from build123d import *

# Parameters (mm, degrees)
F2_R = 0.99999


# Not quite as in the source:
# - a fillet or chamfer is up to 0.001 mm smaller than in the source, because OpenCascade refuses the exact size


with BuildPart() as f1:
    # F0 (on Front) → F1 (revolve)
    with BuildSketch(Plane.XZ):
        with BuildLine():
            Line((-64.5, 52), (-65.5, 52))
            Line((-65.5, 52), (-65.5, 73))
            Line((-65.5, 73), (-67.5, 73))
            Line((-67.5, 73), (-67.5, 50))
            Line((-67.5, 50), (-66.1449700482, 50))
            ThreePointArc((-66.1449700482, 50), (-53.4398255255, 22.2737739938), (-30, 2.761242502))
            Line((-30, 2.761242502), (-30, -2))
            Line((-30, -2), (0, -2))
            Line((0, -2), (0, 0))
            Line((0, 0), (-28, 0))
            Line((-28, 0), (-28, 4))
            ThreePointArc((-28, 4), (-51.9728387009, 23.6482580712), (-64.5, 52))
        make_face()
    revolve(axis=Axis((0, 0, -1), (0, 0, -1)))

    # F2 (radius 1 in the source; OpenCascade refuses exactly that, so slightly less here)
    f2_edges = [f1.edges().sort_by_distance(p)[0] for p in [
        (67.5, 0, 73),
        (65.5, 0, 73),
        (67.5, 0, 50),
        (30, 0, -2),
    ]]
    fillet(f2_edges, radius=F2_R)


solid = f1.part
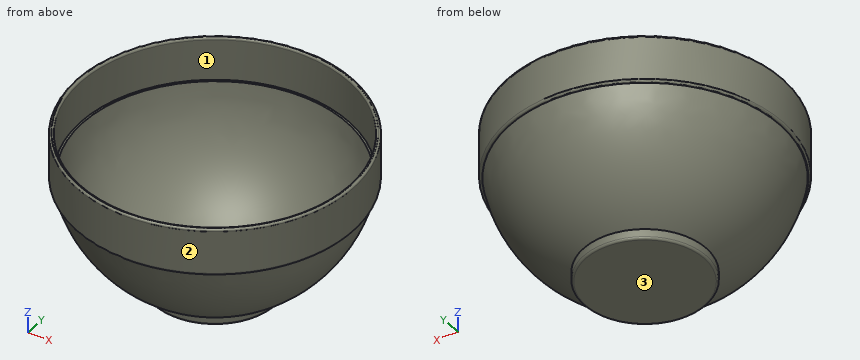
Here's how the part is built. I have some questions about the finished solid (model axes, mm). Face numbers are marked on the shaded views. Give positions to 0.01 mm unless a question says otherwise; leave off trailing zeros. Loops run counter-clockwise (first coordinate to the right, second up) from the corner with the lowest first, then second, coordinate; pieces in that order, holes last. Notation, with made-up numbers: (71.25, 29) -> (80.25, 29) arc R26 cw to (80.25, 62) -> close; hole circle Ø2 at (17, 24.25). An arc over 180 degrees is marked (long way). Answer as a JSON object with one key per item and string values. Group by question number.
Item 1: Imagine slicing it at A-A on z = 59.5. Write out the boundary of the cut face in (x, y).
Item 2: Will these pins go through, and if not, where does the flat tip stop? pin 1 (6 mm diameter, centred on x = -36, z = 52, fed in from -Y); pin 2 (10 mm diameter, centred on x = -14, z = 13, fed in from +Y); pin 3 (6 mm diameter, centred on y = 38.5, z = 38.5, fed in from +X).
Item 3: Thinking about a two-plate mould opening in Y: for the marked faces 1, 2 and 3, which applies, pulls with the +Y half, pulls with the -Y half, needs draft (parallel to the pull), parting line crosses it, or undercut?
Item 4: I need wall thicknesses on L1, parallel to Y at x = 0, z = 2; L2, parallel to Y at x = 0.5, z = 36.5; L3, parallel to X at y = 22, z = 34.5. Which ranges of each line are inside material? Lowest first, please.
Answer list:
{
 "1": {"outline": "circle Ø135 at (0, 0); hole circle Ø131 at (0, 0)"},
 "2": {"pin 1": "stops at y = -58.88", "pin 2": "stops at y = 48.08", "pin 3": "stops at x = 52.08"},
 "3": {"face 1": "undercut", "face 2": "parting line crosses it", "face 3": "needs draft"},
 "4": {"L1": "y = -30 to -28, 28 to 30", "L2": "y = -61.83 to -59.64, 59.64 to 61.83", "L3": "x = -56.8 to -54.41, 54.41 to 56.8"}
}
